Read the model definition and answer for the solid it produces. Units are mm, in the model's axes. Face numbers are marked on the shaded views. A direction names the side the tool comes from. Coordinates: 2 decimals unless noted, no trailing zeros. Loops run counter-clockwise (first coordinate to the right, second up) from the corner with the lowest first, then second, coordinate; pieces in that order, holes last. Notation, with made-up numbers: (13, 76) -> (49, 76) arc R24 cw to (49, 108) -> close; hole circle Ø2 at (33.5, 84.5). An arc over 180 degrees is marked (long way). Answer as a JSON object with one key per item and string values. Group by question number.
Q1. Determine the mould class of the marked faces 1, 2, 3 and 4 for opening direction X: released by +X, released by -X, zero draft, split by the parting line, or undercut.
Q2. For the marked faces 5 and 6, determine the directions among +Z, -Z, +X, -X, +Y, -Y from which every point of the face is accessible in a straight line to the end or side of a thin tool.
Q3. The part is cut by section B-B on y = 82. Write down the section's boundary in (x, z) (3 decimals).
Q4. The part is cut by section D-D on x = 52.5. Write down the section's boundary in (y, z) (3 decimals).
Q5. Straight lines are drawn through the part: line 1 along X through (y, z) = (123.5, 15.5); line 2 along X through (y, z) = (123, 0) (3 decimals); line 3 along Z through (x, y) = (19, 84.5) (3 decimals). For each, find the intervals that lie inside material, in ascending order. Write a range as [from, to].
Q6. The part is cut by section A-A on x = 0. Write down the section's boundary in (y, z) (3 decimals), and give its area (3 significant figures).
Q7. Each of these flat-tipped pins is pushed along its axis until it touches: P1, Ø20, axis at x = -27, z = -13, coming from the -Y side; P2, Ø5.5, axis at x = 0, z = 0, coming from the -Y side; P3, Ø7, axis at x = -1, z = -2, coming from the +Y side. Where does it stop, or does it pass through?
Q8. The part is cut by section C-C on z = 11.5. Write down the section's boundary in (x, y), and give its area (3 significant figures).
from build123d import *

# Parameters (mm, degrees)
SKETCH1_W           = 177.8
SKETCH1_H           = 254
BOSS_EXTRUDE1_DEPTH = 36.445
SHELL1_T            = 3
SKETCH2_R           = 22
CUT_EXTRUDE1_DEPTH  = 3
SKETCH3_R           = 5
CUT_EXTRUDE2_DEPTH  = 3
SKETCH12_W          = 12
SKETCH12_H          = 66.89
BOSS_EXTRUDE5_DEPTH = 6
SKETCH10_R          = 4.525
CUT_EXTRUDE8_DEPTH  = 6
SKETCH13_W          = 174.8
SKETCH13_H          = 69.89
SKETCH13_W_2        = 171.8
SKETCH13_H_2        = 66.89
BOSS_EXTRUDE6_DEPTH = 10
SKETCH14_W          = 175.3
SKETCH14_H          = 70.39
SKETCH14_W_2        = 171.8
SKETCH14_H_2        = 66.89
CUT_EXTRUDE9_DEPTH  = 25
SKETCH17_W          = 171.8
SKETCH17_H          = 66.89
BOSS_EXTRUDE7_DEPTH = 2
SKETCH15_R          = 8.05
CUT_EXTRUDE10_DEPTH = 5
SKETCH18_R          = 2.875
CUT_EXTRUDE11_DEPTH = 4.7
FILLET1_R           = 1.5


with BuildPart() as part:
    # Sketch1 → Boss-Extrude1 (new, symmetric)
    with BuildSketch(Plane.XY):
        Rectangle(SKETCH1_W, SKETCH1_H)
    extrude(amount=BOSS_EXTRUDE1_DEPTH, both=True)

    # Shell1 (no face opened: a closed hollow body)
    add(offset(amount=-SHELL1_T, mode=Mode.PRIVATE), mode=Mode.SUBTRACT)

    # Sketch2 → Cut-Extrude1 (cut)
    with BuildSketch(Plane(origin=(0, 0, 33.445), x_dir=(-1, 0, 0), z_dir=(0, 0, -1))):
        with Locations((0, -4)):
            Circle(SKETCH2_R)
    extrude(amount=-CUT_EXTRUDE1_DEPTH, mode=Mode.SUBTRACT)

    # Sketch3 → Cut-Extrude2 (cut)
    with BuildSketch(Plane.XY.offset(-33.445)):
        with Locations((-20.9, 34)):
            Circle(SKETCH3_R)
    extrude(amount=-CUT_EXTRUDE2_DEPTH, mode=Mode.SUBTRACT)

    # Sketch12 → Boss-Extrude5 (add)
    with BuildSketch(Plane.XZ.offset(-124)):
        Rectangle(SKETCH12_W, SKETCH12_H)
    extrude(amount=BOSS_EXTRUDE5_DEPTH)

    # Sketch10 → Cut-Extrude8 (cut)
    with BuildSketch(Plane(origin=(0, 127, 0), x_dir=(1, 0, 0), z_dir=(0, 1, 0))):
        with Locations(Location((0, 0, 0), (0, 0, 270))):
            Circle(SKETCH10_R)
    extrude(amount=-CUT_EXTRUDE8_DEPTH, mode=Mode.SUBTRACT)


with BuildPart() as body_2:
    # Split2: the piece on the far side of the plane
    add(part.part)
    split(bisect_by=Plane.ZX.offset(52), keep=Keep.BOTTOM)

    # Sketch13 → Boss-Extrude6 (add)
    with BuildSketch(Plane(origin=(0, 52, 0), x_dir=(1, 0, 0), z_dir=(0, 1, 0))):
        Rectangle(SKETCH13_W, SKETCH13_H)
        Rectangle(SKETCH13_W_2, SKETCH13_H_2, mode=Mode.SUBTRACT)
    extrude(amount=BOSS_EXTRUDE6_DEPTH)

    # Sketch17 → Boss-Extrude7 (add)
    with BuildSketch(Plane(origin=(0, -124, 0), x_dir=(1, 0, 0), z_dir=(0, 1, 0))):
        Rectangle(SKETCH17_W, SKETCH17_H)
    extrude(amount=BOSS_EXTRUDE7_DEPTH)

    # Sketch15 → Cut-Extrude10 (cut)
    with BuildSketch(Plane.XZ.offset(127)):
        with Locations(Location((0, 0, 0), (0, 0, 270))):
            Circle(SKETCH15_R)
    extrude(amount=-CUT_EXTRUDE10_DEPTH, mode=Mode.SUBTRACT)

    # Sketch18 → Cut-Extrude11 (cut)
    with BuildSketch(Plane.XZ.offset(127)):
        with Locations(Location((-7.778174593, 7.778174593, 0), (0, 0, 270))):
            Circle(SKETCH18_R)
        with Locations(Location((7.778174593, 7.778174593, 0), (0, 0, 270))):
            Circle(SKETCH18_R)
        with Locations(Location((7.778174593, -7.778174593, 0), (0, 0, 270))):
            Circle(SKETCH18_R)
        with Locations(Location((-7.778174593, -7.778174593, 0), (0, 0, 270))):
            Circle(SKETCH18_R)
    extrude(amount=-CUT_EXTRUDE11_DEPTH, mode=Mode.SUBTRACT)


with BuildPart() as part_1:
    add(part.part)

    # Split2
    split(bisect_by=Plane.ZX.offset(52), keep=Keep.TOP)

    # Sketch14 → Cut-Extrude9 (cut)
    with BuildSketch(Plane.XZ.offset(-52)):
        Rectangle(SKETCH14_W, SKETCH14_H)
        Rectangle(SKETCH14_W_2, SKETCH14_H_2, mode=Mode.SUBTRACT)
    extrude(amount=-CUT_EXTRUDE9_DEPTH, mode=Mode.SUBTRACT)

    # Fillet1
    fillet1_edges = [part_1.edges().sort_by_distance(p)[0] for p in [
        (0, 127, -4.525),
    ]]
    fillet(fillet1_edges, radius=FILLET1_R)


solid = part_1.part
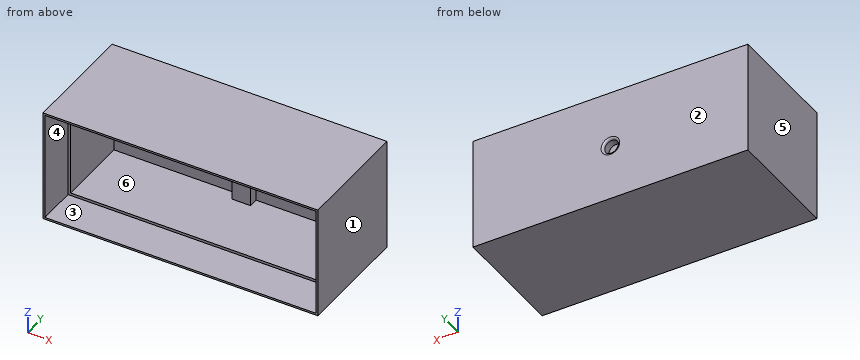
Final values:
{
 "1": {"face 1": "released by +X", "face 2": "zero draft", "face 3": "undercut", "face 4": "undercut"},
 "2": {"face 5": "+Z, -Z, -X, +Y, -Y", "face 6": "-Y"},
 "3": {"outline": "(-88.9, -36.445) -> (88.9, -36.445) -> (88.9, 36.445) -> (-88.9, 36.445) -> close; hole (-85.9, -33.445) -> (85.9, -33.445) -> (85.9, 33.445) -> (-85.9, 33.445) -> close"},
 "4": {"outline": "(52, -36.445) -> (127, -36.445) -> (127, 36.445) -> (52, 36.445) -> (52, 35.195) -> (77, 35.195) -> (77, 33.445) -> (124, 33.445) -> (124, -33.445) -> (77, -33.445) -> (77, -35.195) -> (52, -35.195) -> close"},
 "5": {"line 1": "x = [-88.9, -85.9], [-6, 6], [85.9, 88.9]", "line 2": "x = [-88.9, -85.9], [-6, -4.525], [4.525, 6], [85.9, 88.9]", "line 3": "z = [-36.445, -33.445], [33.445, 36.445]"},
 "6": {"outline": "(52, -36.445) -> (127, -36.445) -> (127, -6.025) arc R1.5 ccw to (125.5, -4.525) -> (121, -4.525) -> (121, 4.525) -> (125.5, 4.525) arc R1.5 ccw to (127, 6.025) -> (127, 36.445) -> (52, 36.445) -> (52, 35.195) -> (77, 35.195) -> (77, 33.445) -> (118, 33.445) -> (118, -33.445) -> (77, -33.445) -> (77, -35.195) -> (52, -35.195) -> close", "area": "909 mm2"},
 "7": {"P1": "stops at y = 124", "P2": "stops at y = 118", "P3": "stops at y = 126.97"},
 "8": {"outline": "(-88.9, 52) -> (-87.65, 52) -> (-87.65, 77) -> (-85.9, 77) -> (-85.9, 124) -> (-6, 124) -> (-6, 118) -> (6, 118) -> (6, 124) -> (85.9, 124) -> (85.9, 77) -> (87.65, 77) -> (87.65, 52) -> (88.9, 52) -> (88.9, 127) -> (-88.9, 127) -> close", "area": "950 mm2"}
}
